from build123d import *

# Parameters (mm, degrees)
BOSS_EXTRUDE1_DEPTH = 6.35
SKETCH3_W           = 19.05
SKETCH3_H           = 6.35
CUT_EXTRUDE1_DEPTH  = 83.611035128


with BuildPart() as part:
    # Sketch1 → Boss-Extrude1 (new body)
    with BuildSketch(Plane.XY):
        Polygon((-25.4, -3.175), (25.4, -3.175), (25.4, 3.175), (31.75, 3.175), (31.75, 9.525), (38.1, 9.525), (38.1, 60.325), (31.75, 60.325), (31.75, 66.675), (25.4, 66.675), (25.4, 73.025), (-25.4, 73.025), (-25.4, 66.675), (-31.75, 66.675), (-31.75, 60.325), (-38.1, 60.325), (-38.1, 9.525), (-31.75, 9.525), (-31.75, 3.175), (-25.4, 3.175), align=None)
    extrude(amount=BOSS_EXTRUDE1_DEPTH)

    # Sketch3 → Cut-Extrude1 (cut, through all)
    with BuildSketch(Plane.XY.offset(6.35)):
        with Locations((28.575, 57.15)):
            Rectangle(SKETCH3_W, SKETCH3_H)
        with Locations((-28.575, 57.15)):
            Rectangle(SKETCH3_W, SKETCH3_H)
    extrude(amount=-CUT_EXTRUDE1_DEPTH, mode=Mode.SUBTRACT)


solid = part.part
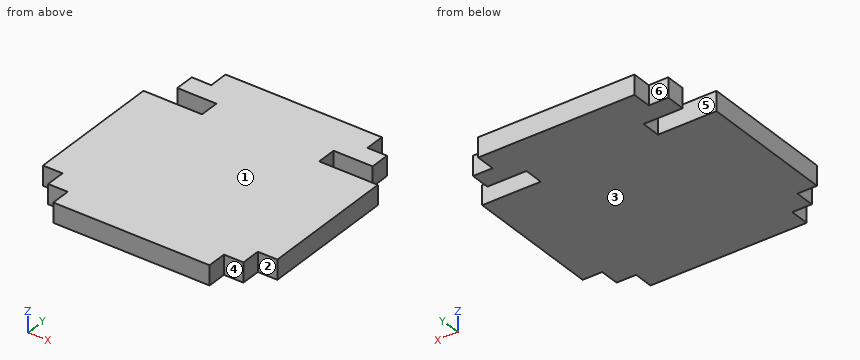
Could you check a few things on this model? Use its own coordinates, in mm. Face numbers are marked on the shaded views. A direction names the side the tool comes from. Coordinates: 2 decimals unless noted, no trailing zeros. Write each loop counter-clockwise with the first axis right and the second up, starting at its lowest first coordinate (ties: lowest second). Pieces come first, ordered by that corner, then holes. Notation, with made-up numbers: (-12, 66.25) - (13, 66.25) arc R20 ccw to (13, 76.25) - close; hole circle Ø10 at (87.25, 68.5). An arc over 180 degrees is marked (long way). Put each result on its own line as item: value. Start each with the question number.
Q1. I want a section at A-A on x = -30. Write out the boundary of the cut face in (y, z) (3 decimals).
Q2. I'm going to push flat-ended pins straight in: P1, Ø3, axis at x = -34, z = 3.5, coming from the -Y side (3 decimals); P2, Ø1.9, axis at y = 0.5, z = 2, coming from the +X side; P3, Ø1.9, axis at y = 56.5, z = 2, coming from the -X side. Where does each tip first touch, or does it pass through?
Q3. Thinking about a two-plate mould opening in Y: for the marked faces 3, 4, 5 and 6, which applies, pulls with the +Y half, pulls with the -Y half, needs draft (parallel to the pull), parting line crosses it, or undercut?
Q4. Please list where these lines run through material, in increasing order: L1, parallel to Y at x = -31.5, z = 1.25 (3 decimals); L2, parallel to Y at x = -21.5, z = 5 (3 decimals); L3, parallel to X at y = 2.5, z = 6.
Q5. Which directions (+Z, -Z, +X, -X, +Y, -Y) give clear straight access to the entire face, cutting with the end or side of a thin tool? Please do the marked faces 1 and 2.
Q6. I want a section at B-B on z = 4. Write out the boundary of the cut face in (x, y) (3 decimals).
Checks:
1. outline: (3.175, 0) - (53.975, 0) - (53.975, 6.35) - (3.175, 6.35) - close; (60.325, 0) - (66.675, 0) - (66.675, 6.35) - (60.325, 6.35) - close
2. P1: y = 9.525
2. P2: x = 25.4
2. P3: x = -19.05
3. face 3: needs draft
3. face 4: pulls with the -Y half
3. face 5: undercut
3. face 6: pulls with the +Y half
4. L1: 3.175 to 53.975, 60.325 to 66.675
4. L2: -3.175 to 53.975, 60.325 to 73.025
4. L3: -25.4 to 25.4
5. face 1: +Z, +X, -X, +Y, -Y
5. face 2: +Z, -Z, +X, -Y
6. outline: (-38.1, 9.525) - (-31.75, 9.525) - (-31.75, 3.175) - (-25.4, 3.175) - (-25.4, -3.175) - (25.4, -3.175) - (25.4, 3.175) - (31.75, 3.175) - (31.75, 9.525) - (38.1, 9.525) - (38.1, 53.975) - (19.05, 53.975) - (19.05, 60.325) - (31.75, 60.325) - (31.75, 66.675) - (25.4, 66.675) - (25.4, 73.025) - (-25.4, 73.025) - (-25.4, 66.675) - (-31.75, 66.675) - (-31.75, 60.325) - (-19.05, 60.325) - (-19.05, 53.975) - (-38.1, 53.975) - close
